Can you work these out from the model? Positions are in its coordinate system, mm. A direction names the side the tool comes from. Round coordinates to 2 decimals unless told otherwise and drop trailing zeros. Order: outer loops, then holes, each group sorted by start corner. A loop starts at its lowest first (then second) coordinate and runs counter-clockwise, first axis right, second up. Notation, with made-up numbers: M -10.75,72.25 L 28.25,72.25 A28 ccw 28.25,91.25 Z; hole C 46.25,82.25 d11. An arc over 180 degrees is marked long. Answer as a JSON object with one key per item and string values. Group by question number.
from build123d import *

# Parameters (mm, degrees)
SKETCH1_W           = 76
SKETCH1_H           = 4
SKETCH2_W           = 19
SKETCH2_H           = 19
BOSS_EXTRUDE1_DEPTH = 6


with BuildPart() as part:
    # Sketch1 → Revolve1 (revolve)
    with BuildSketch(Plane.XY, mode=Mode.PRIVATE) as revolve1_sk:
        with Locations((38, 2)):
            Rectangle(SKETCH1_W, SKETCH1_H)
    revolve(revolve1_sk.sketch.rotate(Axis((0, 0, 0), (1, 0, 0)), 90), axis=Axis((0, 0, 0), (1, 0, 0)))  # turned: the seam where the file's is

    # Sketch2 → Boss-Extrude1 (add)
    with BuildSketch(Plane.ZY):
        Rectangle(SKETCH2_W, SKETCH2_H)
    extrude(amount=BOSS_EXTRUDE1_DEPTH)


solid = part.part
Item 1: Suppose I cut it at C-C, the plane x = 13.5. Write out the boundary of the cut face in (y, z).
Item 2: On a 3-axis mill with a long thin cutter (end or side, diameter ignored), from which of +Z, -Z, +X, -X, +Y, -Y can I reach the whole of each face in a straight line? I mean faces 1 (the face through (-3, 0, -9.5)), 2 (the face through (0, 0.1, -4.4)). Say none if no direction works.
Item 3: I need wall thicknesses on line 1 (X direction, y = 4, z = 3.75); line 2 (Y direction, x = 27.5, z = 2.75); line 3 (Y direction, x = 18, z = -2.25). Which ranges of each line are inside material? Lowest first, please.
Item 4: Suppose I cut it at D-D, the plane z = -5.25. Write out the boundary of the cut face in (x, y).
Item 5: I'm going to push flat-ended pins straight in: pin 1 Ø8 at (x, z) = (15, 2.5) entering from +Y; pin 2 Ø3 at (x, z) = (47.5, -4.5) entering from +Y; pin 3 Ø3 at (x, y) = (21, -2) entering from -Z. Where does each tip first touch, or does it pass through?
Item 6: Suppose I cut it at A-A, the plane y = 0. Write out the boundary of the cut face in (x, z), and give its area (3 significant figures).
Computed:
{
 "1": {"outline": "C 0,0 d8"},
 "2": {"face 1": "-Z, +X, -X, +Y, -Y", "face 2": "+X"},
 "3": {"line 1": "x = -6 to 0", "line 2": "y = -2.9 to 2.9", "line 3": "y = -3.31 to 3.31"},
 "4": {"outline": "M -6,-9.5 L 0,-9.5 L 0,9.5 L -6,9.5 Z"},
 "5": {"pin 1": "stops at y = 4", "pin 2": "stops at y = 2.65", "pin 3": "stops at z = -3.97"},
 "6": {"outline": "M -6,-9.5 L 0,-9.5 L 0,-4 L 76,-4 L 76,4 L 0,4 L 0,9.5 L -6,9.5 Z", "area": "722 mm^2"}
}
